Part print with two shaded views. Sizes in mm from the minimum x, y, z corner. A direction names the side the tool comes from. Coordinates: 2 decimals unless noted, no trailing zeros. Loops run counter-clockwise (first coordinate to the right, second up) from the corner with the lowest first, then second, coordinate; pieces in that order, holes last.
(1) Slice it at A-A (y = 16). Give the cut face in (x, z), and give its area (3 significant figures).
(2) Slice it at C-C (z = 17.25). Give the cut face in (x, y).
(3) Flat gauge pins, fed straight in: P1, Ø1.5, axis at x = 26.5, y = 4.5, coming from the -Z side; P2, Ø3, axis at x = 17, z = 14.5, coming from the +Y side; P3, Ø12, axis at x = 19.5, z = 17.5, coming from the +Y side; P4, Ø4, axis at x = 13.5, y = 22, coming from the -Z side. Where does each tip first touch, or does it go through?
(4) Wall check: L1, parallel to Y at x = 23.25, z = 16.25; L2, parallel to Y at x = 27.5, z = 17; L3, parallel to Z at x = 7.25, y = 11. Give the ranges that are in metal, low to high.
(5) Two-plate mould, pull along Z, no slides. Class the marked faces 1, 2, 3 and 4: pulls with the +Z half, pulls with the -Z half, needs draft (parallel to the pull), parting line crosses it, or undercut.
(6) Slice it at B-B (x = 7.75). Give the cut face in (y, z).
(7) Tool access for the marked faces 5, 6 and 7: list every direction of +Z, -Z, +X, -X, +Y, -Y with a clear straight run to the whole face (end or side of a thin tool).
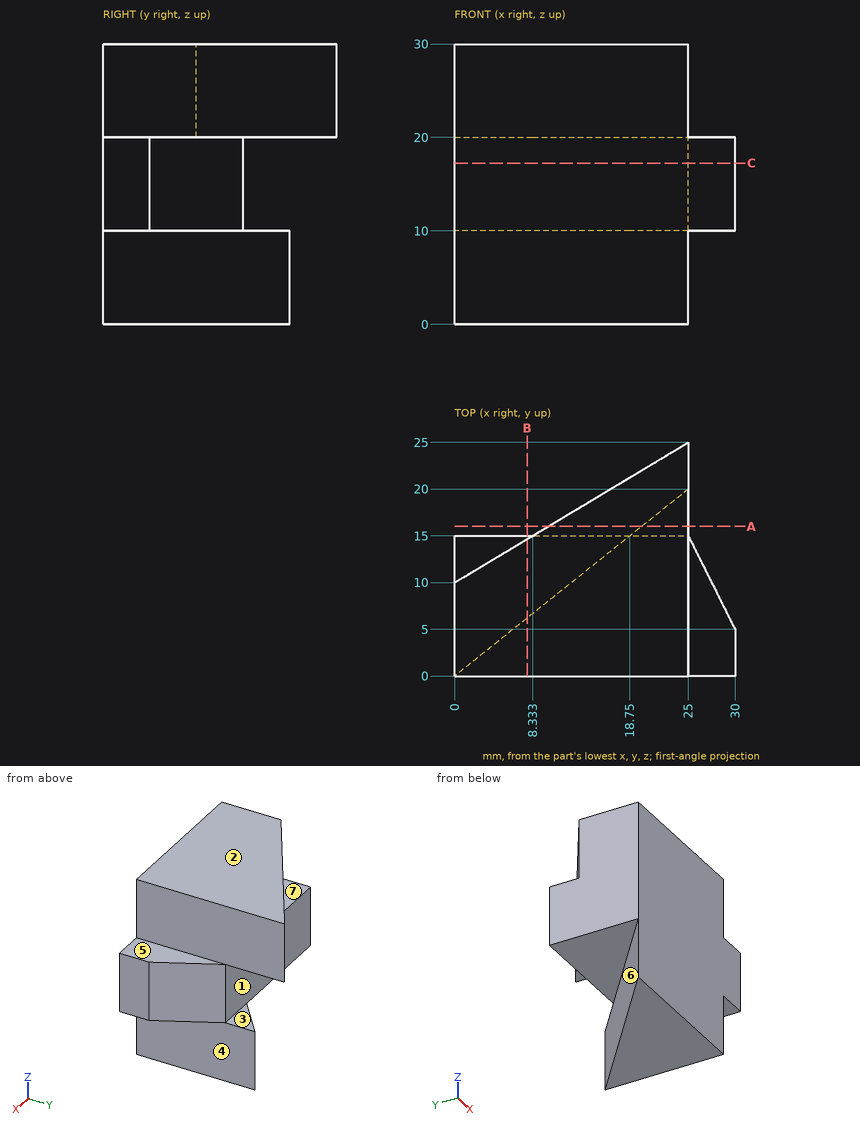
Response values:
1. outline: (10, 20) - (25, 20) - (25, 30) - (10, 30) - close; (20, 0) - (25, 0) - (25, 10) - (20, 10) - close
1. area: 200 mm2
2. outline: (0, 0) - (30, 0) - (30, 5) - (25, 15) - (0, 15) - close
3. P1: stops at z = 10
3. P2: stops at y = 15
3. P3: stops at y = 24.97
3. P4: passes through
4. L1: y = 0 to 15
4. L2: y = 0 to 10
4. L3: z = 10 to 30
5. face 1: undercut
5. face 2: pulls with the +Z half
5. face 3: undercut
5. face 4: needs draft
6. outline: (0, 0) - (6.2, 0) - (6.2, 10) - (15, 10) - (15, 20) - (14.65, 20) - (14.65, 30) - (0, 30) - close
7. face 5: +Z, +X, +Y, -Y
7. face 6: -Z, -X, +Y
7. face 7: +Z, -X, +Y
